Answer from the drawing. Dimensions are ordinates in mm from the lowest x, y and z of the part. A direction names the side the tool comes from. Coordinates: 2 decimals unless noted, no trailing zeros. Order: outer loops, then holes, each group sorted by start corner. A loop starts at its lowest first (then second) coordinate and runs counter-clockwise, first axis right, second up. Notation, with made-up numbers: (43.5, 49.25) -> (79.5, 49.25) arc R23 ccw to (79.5, 87.25) -> close; hole circle Ø10 at (70, 6.25). An arc over 180 degrees is marked (long way). Answer as a JSON object with one key per item and string values. Group by question number.
1) Determine the mould class of the marked faces 3, 4 and 5 for opening direction X: released by +X, released by -X, zero draft, split by the parting line, or undercut.
2) Section D-D on z = 23 is taken. Determine the outline of the cut face in (x, y).
3) A tool of negligible diameter and unlimited length cuts with its end or side. For the marked faces 1 and 2, from which of +Z, -Z, +X, -X, +Y, -Y can it reach the whole face along a straight path? Write none if from no direction.
4) Section A-A on z = 17.5 is taken. Determine the outline of the cut face in (x, y), and give its area (3 significant figures).
5) Given pin 1 (4 mm diameter, centred on x = 14.5, y = 5, fed in from -Z); pin 2 (5 mm diameter, centred on x = 10, y = 2, fed in from +Z); pin 3 (4 mm diameter, centred on x = 17.5, z = 30, fed in from -Y); pin 4 (8 mm diameter, centred on x = 30, z = 28, fed in from +Y), each flat-ended and moving along its own axis, determine where each tip first touches the part or whether it passes through.
6) Consider L1, parallel to Z at x = 17.5, y = 4.3; L2, parallel to Z at x = 17.5, y = 7.25; L3, parallel to X at y = 3.25, z = 17.5. Determine where each line is inside the solid, lowest interval first.
7) Section B-B on y = 5.25 is taken. Determine the outline of the cut face in (x, z), and give its area (3 significant figures).
8) Section C-C on x = 9 is taken. Determine the outline of the cut face in (y, z), and give its area (3 significant figures).
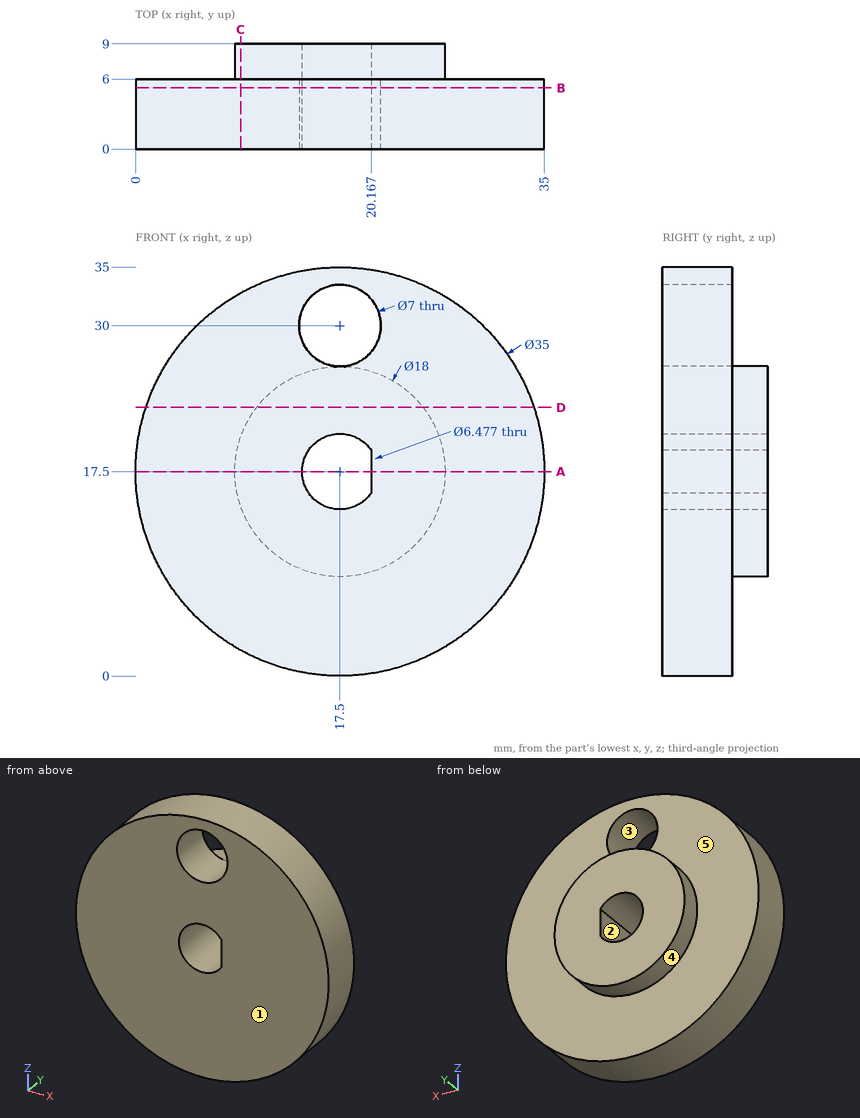
Worked answers:
{
 "1": {"face 3": "undercut", "face 4": "split by the parting line", "face 5": "zero draft"},
 "2": {"outline": "(0.89, 0) -> (34.11, 0) -> (34.11, 6) -> (24.62, 6) -> (24.62, 9) -> (10.38, 9) -> (10.38, 6) -> (0.89, 6) -> close"},
 "3": {"face 1": "+Z, -Z, +X, -X, -Y", "face 2": "+Y, -Y"},
 "4": {"outline": "(0, 0) -> (14.26, 0) -> (14.26, 9) -> (8.5, 9) -> (8.5, 6) -> (0, 6) -> close; (20.17, 0) -> (35, 0) -> (35, 6) -> (26.5, 6) -> (26.5, 9) -> (20.17, 9) -> close", "area": "211 mm²"},
 "5": {"pin 1": "stops at z = 0.03", "pin 2": "stops at z = 34.27", "pin 3": "passes through", "pin 4": "stops at y = 6"},
 "6": {"L1": "z = 0 to 14.26, 20.74 to 26.5, 33.5 to 35", "L2": "z = 8.5 to 14.26, 20.74 to 26.5", "L3": "x = 0 to 14.26, 20.17 to 35"},
 "7": {"outline": "circle Ø35 at (17.5, 17.5); hole circle Ø7 at (17.5, 30); hole (20.17, 15.66) -> (20.17, 19.34) arc R3.24 ccw (long way) to start", "area": "892 mm²"},
 "8": {"outline": "(0, 2.2) -> (6, 2.2) -> (6, 14.54) -> (9, 14.54) -> (9, 20.46) -> (6, 20.46) -> (6, 32.8) -> (0, 32.8) -> close", "area": "201 mm²"}
}
